For this review, take the finished solid that the model builds, in its own axes (mm). Face numbers are marked on the shaded views. A direction names the side the tool comes from. Coordinates: 2 decimals unless noted, no trailing zeros. Order: outer loops, then holes, each group sorted by start corner. A loop starts at its lowest first (then second) coordinate and runs counter-clockwise, first axis right, second up.
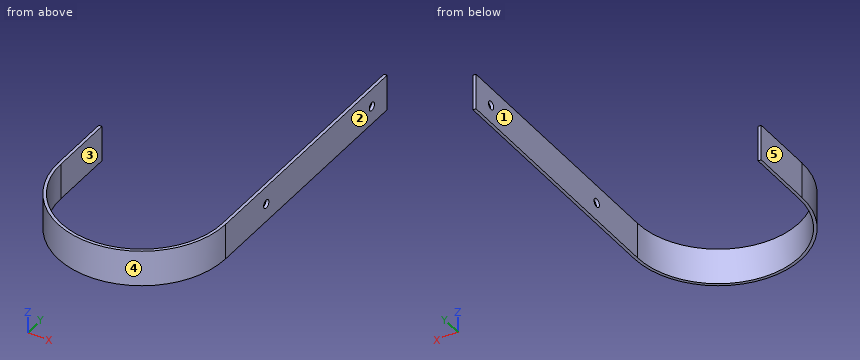
Autodesk Inventor part; units mm, degrees
ref_plane "YZ Plane" through (0, 0, 0) normal (1, 0, 0) x (0, 1, 0)
ref_plane "XZ Plane" through (0, 0, 0) normal (0, 1, 0) x (-1, 0, 0)
ref_plane "XY Plane" through (0, 0, 0) normal (0, 0, 1) x (1, 0, 0)
sketch "Sketch1" plane through (0, 0, 0) normal (0, 1, 0) x (-1, 0, 0)
  line L0 (152.4, -9.525) -> (-152.4, -9.525)
  line L1 (-152.4, -9.525) -> (-152.4, 9.525)
  line L2 (-152.4, 9.525) -> (152.4, 9.525)
  line L3 (152.4, 9.525) -> (152.4, -9.525)
  line L4 (152.4, -9.525) -> (-152.4, 9.525) construction
  line L5 (-152.4, -9.525) -> (152.4, 9.525) construction
  point P0 (0, 0)
  dimension "d0" = 19.05
  dimension "d1" = 304.8
extrude "Extrusion1" add sketch "Sketch1" along normal blind 1.5875
sketch "Sketch2" plane through (0, 1.5875, 0) normal (0, 1, 0) x (1, 0, 0)
  line L0 (152.4, -9.525) -> (152.4, 9.525)
  line L1 (50.8, 36.3839) -> (50.8, -48.8029) construction
  line L2 (-50.8, 37.7294) -> (-50.8, -44.9073)
  line L3 (152.4, 9.525) -> (-152.4, 9.525)
  line L4 (-152.4, 9.525) -> (-152.4, -9.525)
  line L5 (-152.4, -9.525) -> (152.4, -9.525)
  line L6 (152.4, -9.525) -> (152.4, 9.525)
  line L7 (-152.4, 9.525) -> (50.8, -9.525) construction
  line L8 (50.8, 9.525) -> (-152.4, -9.525) construction
  point P0 (0, 0)
  point P1 (-50.8, 0)
  dimension "d4" = 101.6
bend part "Bend Part2" radius 42.8509 angle 180 line through (-50.8, 1.5875, -37.7294) along (0, 0, 1) centre toward (0, 1, 0) moving side (1, 0, 0) both sides yes
sketch "Sketch3" plane through (-6.3616, 44.4384, -9.525) normal (1, 0, 0) x (0, 0, -1)
  line L0 (-19.05, 0) -> (0, 0)
  line L1 (0, 135.89) -> (-19.05, 135.89)
  line L2 (-19.05, 135.89) -> (-19.05, 0)
  circle A0 centre (-9.525, 123.19) radius 2.2225
  line L3 (-19.05, 0) -> (0, 135.89) construction
  line L4 (-19.05, 135.89) -> (0, 0) construction
  line L5 (-9.525, 0) -> (-9.525, 135.89) construction
  circle A1 centre (-9.525, 34.29) radius 2.2225
  point P0 (-9.525, -44.4384)
  dimension "d9" = 4.445
  dimension "d10" = 12.7
  dimension "d13" = 88.9
extrude "Extrusion2" cut sketch "Sketch3" against normal blind 1.5875
properties part number "side guard" material "Polycarbonate, Clear"
1. To check wall thickness, follow L1, parallel to X at y = 44, z = -0.5; L2, parallel to X at y = 118, z = -5. State the ranges of each line that lie inside material, in increasing order.
Answer below:
L1: x = -95.24 to -93.65, -7.95 to -6.36
L2: x = -7.95 to -6.36
2. Take a section at A-A, the plane z = 0. Give the boundary of the cut face in (x, y), plus the area to 3 significant figures.
Answer below:
outline: (-95.24, 44.44) arc R44.44 ccw to (-6.36, 44.44) - (-6.36, 76.51) - (-7.95, 76.51) - (-7.95, 44.44) arc R42.85 cw to (-93.65, 44.44) - (-93.65, 78.73) - (-95.24, 78.73) - close; (-7.95, 80.95) - (-6.36, 80.95) - (-6.36, 165.41) - (-7.95, 165.41) - close; (-7.95, 169.85) - (-6.36, 169.85) - (-6.36, 180.33) - (-7.95, 180.33) - close
area: 474 mm2
3. The part is to be moulded in two halves that separate along X. For the marked faces 3, 4 and 5, say which applies: +X half, -X half, draft (parallel to the pull), parting line (faces both ways), or undercut.
Answer below:
face 3: undercut
face 4: parting line
face 5: -X half
4. Take a section at D-D, the plane x = -50.8. Give the boundary of the cut face in (y, z) (1 decimal), plus the area to 3 significant figures.
Answer below:
outline: (0, -9.5) - (1.6, -9.5) - (1.6, 9.5) - (0, 9.5) - close
area: 30.2 mm2
5. Machinability: for the marked faces 1 and 2, which of the approach directions +Z, -Z, +X, -X, +Y, -Y give a long, thin tool a straight path to every point of the face, cutting with its end or side? Answer none if there is none.
Answer below:
face 1: +Z, -Z, +Y
face 2: +Z, -Z, +X, +Y, -Y
6. Clearance check with flat-ended pins moving along their axes: pin 1 Ø2 at (x, z) = (-51, -1.5) entering from -Y; pin 2 Ø2.5 at (y, z) = (167.63, 0) entering from -X; pin 3 Ø1 at (x, z) = (-76, 0.5) entering from +Y; pin 4 Ø4 at (y, z) = (105.5, -4) entering from -X. State where each tip first meets the part, or that it passes through.
Answer below:
pin 1: stops at y = 0
pin 2: passes through
pin 3: stops at y = 10.15
pin 4: stops at x = -7.95
7. Take a section at B-B, the plane y = 56. Give the boundary of the cut face in (x, z) (3 decimals), plus the area to 3 significant figures.
Answer below:
outline: (-95.238, -9.525) - (-93.651, -9.525) - (-93.651, 9.525) - (-95.238, 9.525) - close; (-7.949, -9.525) - (-6.362, -9.525) - (-6.362, 9.525) - (-7.949, 9.525) - close
area: 60.5 mm2
8. Take a section at C-C, the plane z = 7.25. Give the boundary of the cut face in (x, y).
Answer below:
outline: (-95.24, 44.44) arc R44.44 ccw to (-6.36, 44.44) - (-6.36, 180.33) - (-7.95, 180.33) - (-7.95, 44.44) arc R42.85 cw to (-93.65, 44.44) - (-93.65, 78.73) - (-95.24, 78.73) - close
